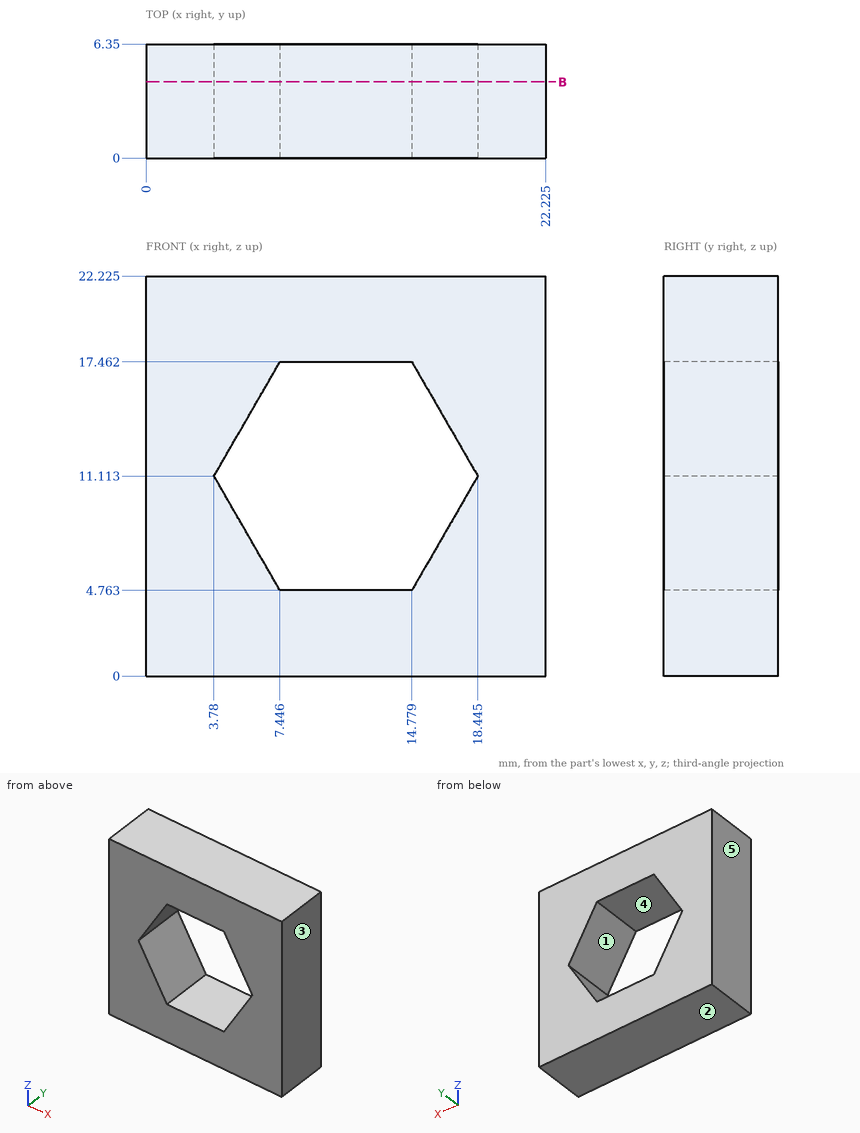
Answer from the drawing. Dimensions are ordinates in mm from the lowest x, y and z of the part. A direction names the side the tool comes from. Round coordinates to 2 decimals unless told otherwise and drop trailing zeros. Write each loop counter-clockwise with the first axis right and the second up, starting at its lowest first coordinate (ties: lowest second). Pieces come first, ordered by that corner, then holes. Notation, with made-up numbers: M 36,-39.75 L 65,-39.75 A4 ccw 65,-33.75 Z; hole C 44.25,41 d11. An arc over 180 degrees is marked long. One line per item, written item: value.
Q1. Find section B-B on y = 4.25. Write down the section's boundary in (x, z) (1 decimal).
Data:
outline: M 0,0 L 22.2,0 L 22.2,22.2 L 0,22.2 Z; hole M 3.8,11.1 L 7.4,4.8 L 14.8,4.8 L 18.4,11.1 L 14.8,17.5 L 7.4,17.5 Z
Q2. Which of the six approach directions +Z, -Z, +X, -X, +Y, -Y give full straight-line access (tool end or side, diameter ignored) to the marked faces 4 and 5?
Data:
face 4: +Y, -Y
face 5: +Z, -Z, -X, +Y, -Y
Q3. Straight lines are drawn through the part: line 1 (Z direction, x = 11.25, y = 4.25) (1 decimal); line 2 (X direction, y = 0.5, z = 12.75) (1 decimal); line 3 (Z direction, x = 16.25, y = 2.25) (1 decimal). For each, find the intervals that lie inside material, in ascending order. Write a range as [from, to].
Data:
line 1: [0, 4.8], [17.5, 22.2]
line 2: [0, 4.7], [17.5, 22.2]
line 3: [0, 7.3], [14.9, 22.2]
Q4. For a pull along Z with two mould halves and no side action, classify the marked faces 1, 2 and 3 as +Z half, -Z half, draft (parallel to the pull), parting line (faces both ways), or undercut.
Data:
face 1: undercut
face 2: -Z half
face 3: draft
